Drawing for the job (mm, zero at the part's lowest x, y, z). Give positions to 0.01 mm unless a question says otherwise; leave off trailing zeros. Loops run counter-clockwise (first coordinate to the right, second up) from the corner with the lowest first, then second, coordinate; pieces in that order, holes last. Notation, with made-up numbers: M -4,87.5 L 44,87.5 A31 cw 44,113.5 Z; hole C 40,60 d10. An arc over 180 degrees is marked long. Answer in a Markdown table with one row per item. Add a question column.
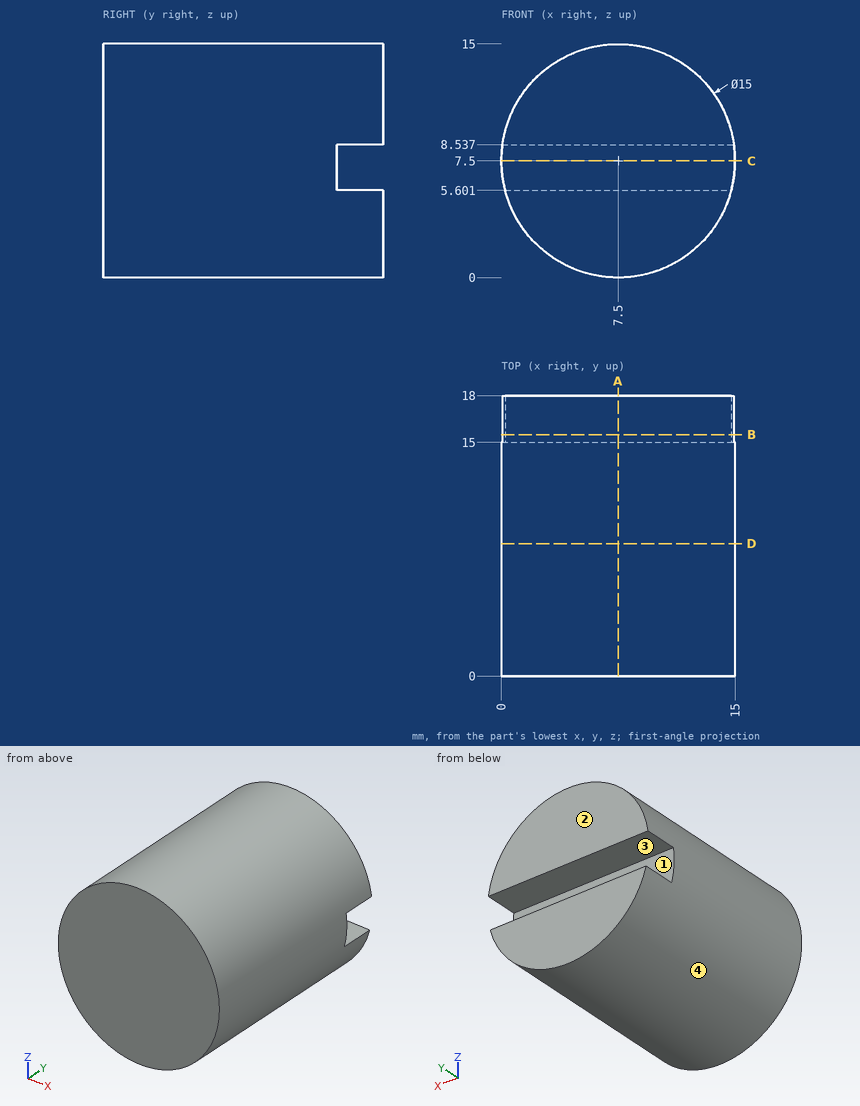
(1) Pull direction Z, two halves, no side cores. Call the marked faces 1, 2, 3 and 4: +Z half, -Z half, draft (parallel to the pull), parting line (faces both ways), or undercut.
(2) Wall check: line 1 (Y direction, x = 1.25, z = 7); line 2 (Z direction, x = 8.75, y = 16.75) (1 decimal); line 3 (Z direction, x = 6.5, y = 10). Give the ranges that are in metal, low to high.
(3) Slice it at B-B, the plane y = 15.5. Give the cut face in (x, z).
(4) Slice it at C-C, the plane z = 7.5. Give the cut face in (x, y), then the cut area to 3 significant figures.
(5) Pin check, flat tips, straight feed: pin 1 (6 mm diameter, centred on y = 13, z = 13.5, fed in from +X); pin 2 (2 mm diameter, centred on y = 10.5, z = 2.5, fed in from +X); pin 3 (4 mm diameter, centred on x = 12, y = 10, fed in from +Z). Stop position of each tip, or through.
(6) Slice it at D-D, the plane y = 8.5. Give the cut face in (x, z).
(7) Slice it at A-A, the plane x = 7.5. Give the cut face in (y, z), then the cut area to 3 significant figures.
Solution:
| question | item | result |
|---|---|---|
| 1 | face 1 | undercut |
| 1 | face 2 | draft |
| 1 | face 3 | undercut |
| 1 | face 4 | parting line |
| 2 | line 1 | 0 to 15 |
| 2 | line 2 | 0.1 to 5.6, 8.5 to 14.9 |
| 2 | line 3 | 0.07 to 14.93 |
| 3 | outline | M 0.07,8.54 L 14.93,8.54 A7.5 ccw Z; M 0.24,5.6 A7.5 ccw 14.76,5.6 Z |
| 4 | outline | M 0,0 L 15,0 L 15,15 L 0,15 Z |
| 4 | area | 225 mm^2 |
| 5 | pin 1 | x = 14.37 |
| 5 | pin 2 | x = 13.84 |
| 5 | pin 3 | z = 14.57 |
| 6 | outline | C 7.5,7.5 d15 |
| 7 | outline | M 0,0 L 18,0 L 18,5.6 L 15,5.6 L 15,8.54 L 18,8.54 L 18,15 L 0,15 Z |
| 7 | area | 261 mm^2 |
